from build123d import *

# Parameters (mm, degrees)
SKETCH1_R           = 2
SKETCH1_R_2         = 12
BOSS_EXTRUDE1_DEPTH = 5
SKETCH2_W           = 32.3
SKETCH2_H           = 3.175
BOSS_EXTRUDE2_DEPTH = 32
CHAMFER1_SIZE       = 3
CUT_EXTRUDE1_DEPTH  = 10
CUT_EXTRUDE2_DEPTH  = 10
BOSS_EXTRUDE3_REACH = 53.634
SKETCH5_W           = 9.21920545
SKETCH5_H           = 4.68574677


with BuildPart() as part:
    # Sketch1 → Boss-Extrude1 (new body)
    with BuildSketch(Plane.XY):
        Polygon((-21.15, -16.907359313), (-21.15, 24.149999999), (-16.15, 24.149999999), (-16.15, 29.149999999), (16.15, 29.149999999), (16.15, 24.149999999), (21.15, 24.149999999), (21.15, -16.907359313), (16.907359313, -21.15), (-16.907359313, -21.15), align=None)
        with Locations((-15.5, 15.5)):
            Circle(SKETCH1_R, mode=Mode.SUBTRACT)
        with Locations((-15.5, -15.5)):
            Circle(SKETCH1_R, mode=Mode.SUBTRACT)
        Circle(SKETCH1_R_2, mode=Mode.SUBTRACT)
        with Locations((15.5, -15.5)):
            Circle(SKETCH1_R, mode=Mode.SUBTRACT)
        with Locations((15.5, 15.5)):
            Circle(SKETCH1_R, mode=Mode.SUBTRACT)
    extrude(amount=BOSS_EXTRUDE1_DEPTH)

    # Sketch2 → Boss-Extrude2 (add)
    with BuildSketch(Plane(origin=(0, 0, 0), x_dir=(-1, 0, 0), z_dir=(0, 0, -1))):
        with Locations((0, 27.562499999)):
            Rectangle(SKETCH2_W, SKETCH2_H)
    extrude(amount=BOSS_EXTRUDE2_DEPTH)

    # Chamfer1
    chamfer1_edges = [part.edges().sort_by_distance(p)[0] for p in [
        (0, 25.974999999, 0),
    ]]
    chamfer(chamfer1_edges, length=CHAMFER1_SIZE)

    # Sketch3 → Cut-Extrude1 (cut)
    with BuildSketch(Plane.XZ.offset(-25.974999999)):
        with BuildLine():
            Line((7.2, -9.25), (7.2, -6))
            ThreePointArc((7.2, -6), (10, -3.2), (12.8, -6))
            Line((12.8, -6), (12.8, -9.25))
            ThreePointArc((12.8, -9.25), (10, -12.05), (7.2, -9.25))
        make_face()
        with BuildLine():
            Line((-12.799999999, -9.25), (-12.799999999, -6))
            ThreePointArc((-12.799999999, -6), (-9.999999999, -3.2), (-7.199999999, -6))
            Line((-7.199999999, -6), (-7.199999999, -9.25))
            ThreePointArc((-7.199999999, -9.25), (-9.999999999, -12.05), (-12.799999999, -9.25))
        make_face()
        with BuildLine():
            Line((12.8, -21.25), (12.8, -24.5))
            ThreePointArc((12.8, -24.5), (10, -27.3), (7.2, -24.5))
            Line((7.2, -24.5), (7.2, -21.25))
            ThreePointArc((7.2, -21.25), (10, -18.45), (12.8, -21.25))
        make_face()
        with BuildLine():
            Line((-7.199999999, -21.25), (-7.199999999, -24.5))
            ThreePointArc((-7.199999999, -24.5), (-9.999999999, -27.3), (-12.799999999, -24.5))
            Line((-12.799999999, -24.5), (-12.799999999, -21.25))
            ThreePointArc((-12.799999999, -21.25), (-9.999999999, -18.45), (-7.199999999, -21.25))
        make_face()
    extrude(amount=-CUT_EXTRUDE1_DEPTH, mode=Mode.SUBTRACT)

    # Sketch4 → Cut-Extrude2 (cut)
    with BuildSketch(Plane.XY.offset(5)):
        Polygon((16.15, 24.149999999), (21.15, 19.149999999), (21.15, 24.149999999), align=None)
        Polygon((-21.15, 24.149999999), (-16.15, 24.149999999), (-21.15, 19.149999999), align=None)
    extrude(amount=-CUT_EXTRUDE2_DEPTH, mode=Mode.SUBTRACT)

    # Boss-Extrude3: up to this plane
    boss_extrude3_end = Plane(origin=(-16.15, 25.974999999, -3), z_dir=(0, -0.7071067811865506, -0.7071067811865445))
    # Sketch5 → Boss-Extrude3 (add, up to the surface)
    with BuildSketch(Plane(origin=(0, 0, -32), x_dir=(-1, 0, 0), z_dir=(0, 0, -1)), mode=Mode.PRIVATE) as boss_extrude3_sk1:
        with Locations((0, 25.974999999)):
            Rectangle(SKETCH5_W, SKETCH5_H)
    boss_extrude3_tool1 = split(extrude(boss_extrude3_sk1.sketch, amount=-BOSS_EXTRUDE3_REACH, mode=Mode.PRIVATE), bisect_by=boss_extrude3_end, keep=Keep.BOTH, mode=Mode.PRIVATE)
    add(boss_extrude3_tool1.solids().sort_by_distance((0, 25.975, -32))[0])


solid = part.part
Here's how the part is built. I have some questions about the finished solid (model axes, mm). A direction names the side the tool comes from. Round coordinates to 2 decimals unless told otherwise and drop trailing zeros. Loops run counter-clockwise (first coordinate to the right, second up) from the corner with the lowest first, then second, coordinate; pieces in that order, holes last. Notation, with made-up numbers: (45.5, 4.25) -> (82.5, 4.25) arc R30 ccw to (82.5, 42.25) -> close; hole circle Ø5 at (74, 66.25). An arc over 180 degrees is marked (long way). Write each question's results on one line, items separated by ' | '.
(1) For faces 1 (the face through (-16.15, 27, -13)), 2 (the face through (4.61, 25, -17)), 3 (the face through (7.2, 28, -23)), which set-ups out of +Z, -Z, +X, -X, +Y, -Y let a thin tool reach every point of the face, with its end or its side?
Worked answers:
face 1: +Z, -Z, -X, +Y | face 2: -Z, +X, -Y | face 3: +Y, -Y
(2) For P1, Ø4.5, axis at x = -15.5, y = 15.5, coming from the -Z side; P2, Ø1.6, axis at y = 27.5, z = -22.5, coming from the -X side; P3, Ø6.5, axis at x = -15.5, y = -15.5, coming from the +Z side; P4, Ø3.5, axis at y = 28.5, z = -23.5, coming from the +X side, each with a flat end and sliding along its axis, tell me the tip position at first contact or that it passes through.
Worked answers:
P1: z = 0 | P2: x = -16.15 | P3: z = 5 | P4: x = 16.15
(3) If we section it at C-C, the plane y = -15.5: List the corners of the cut face in (x, z) for me, then the cut area to 4 significant figures.
Worked answers:
outline: (-21.15, 0) -> (-17.5, 0) -> (-17.5, 5) -> (-21.15, 5) -> close; (-13.5, 0) -> (13.5, 0) -> (13.5, 5) -> (-13.5, 5) -> close; (17.5, 0) -> (21.15, 0) -> (21.15, 5) -> (17.5, 5) -> close | area: 171.5 mm2
(4) If we section it at B-B, the plane z = -8: List the corners of the cut face in (x, y) for me (3 decimals).
Worked answers:
outline: (-16.15, 25.975) -> (-12.8, 25.975) -> (-12.8, 29.15) -> (-16.15, 29.15) -> close; (-7.2, 25.975) -> (-4.61, 25.975) -> (-4.61, 23.632) -> (4.61, 23.632) -> (4.61, 25.975) -> (7.2, 25.975) -> (7.2, 29.15) -> (-7.2, 29.15) -> close; (12.8, 25.975) -> (16.15, 25.975) -> (16.15, 29.15) -> (12.8, 29.15) -> close
(5) If I drill on L1, parallel to Y at x = 15.5, z = 4.05; L2, parallel to Y at x = 15, z = 3; L3, parallel to Y at x = 0, z = 1.7, over which ranges is the centre line in solid material (lowest first)?
Worked answers:
L1: -21.15 to -17.5, -13.5 to 13.5, 17.5 to 29.15 | L2: -21.15 to -17.44, -13.56 to 13.56, 17.44 to 29.15 | L3: -21.15 to -12, 12 to 29.15
(6) If we section it at A-A, the plane x = 0: List the corners of the cut face in (y, z) for me (3 decimals).
Worked answers:
outline: (-21.15, 0) -> (-12, 0) -> (-12, 5) -> (-21.15, 5) -> close; (12, 0) -> (22.975, 0) -> (23.632, -0.657) -> (23.632, -32) -> (29.15, -32) -> (29.15, 5) -> (12, 5) -> close
(7) If we section it at D-D, the plane x = -10: List the corners of the cut face in (y, z) for me (3 decimals), then the cut area to 3 significant figures.
Worked answers:
outline: (-21.15, 0) -> (-6.633, 0) -> (-6.633, 5) -> (-21.15, 5) -> close; (6.633, 0) -> (22.975, 0) -> (25.975, -3) -> (25.975, -3.2) -> (29.15, -3.2) -> (29.15, 5) -> (6.633, 5) -> close; (25.975, -32) -> (29.15, -32) -> (29.15, -27.3) -> (25.975, -27.3) -> close; (25.975, -18.45) -> (29.15, -18.45) -> (29.15, -12.05) -> (25.975, -12.05) -> close | area: 235 mm2
(8) We'd pull the mould along Y, two halves only. Please class faces 4 (the face through (16.15, 27, -13)), 5 (the face through (-11.99, 0.53, 2.46)), 6 (the face through (-18.6, 21.7, 2.6)), 7 (the face through (0.243, 23.496, -0.521)): released by +Y, released by -Y, zero draft, split by the parting line, or undercut.
Worked answers:
face 4: zero draft | face 5: undercut | face 6: released by +Y | face 7: released by -Y
